Autodesk Inventor part; units mm, degrees
ref_plane "YZ Plane" through (0, 0, 0) normal (1, 0, 0) x (0, 1, 0)
ref_plane "XZ Plane" through (0, 0, 0) normal (0, 1, 0) x (-1, 0, 0)
ref_plane "XY Plane" through (0, 0, 0) normal (0, 0, 1) x (1, 0, 0)
sketch "Sketch1" plane through (0, 0, 0) normal (0, 1, 0) x (-1, 0, 0)
  line L0 (0, 0) -> (-30.566, 0)
  line L1 (-30.566, 0) -> (-30.566, -53)
  line L2 (-30.566, -53) -> (0, -53)
  line L3 (0, -53) -> (0, 0)
  dimension "d0" = 30.566
  dimension "d1" = 53
extrude "Extrusion1" add sketch "Sketch1" along normal blind 2
ref_plane "Work Plane1" through (30.566, 0, -23) normal (0, 0, -1) x (-1, 0, 0)
sketch "Sketch2" plane through (30.566, 0, -23) normal (0, 0, -1) x (-1, 0, 0)
  point P0 (30.566, 0)
sketch "Sketch3" plane through (30.566, 0, -53) normal (0, 0, -1) x (-1, 0, 0)
  circle A0 centre (30.566, 0) radius 1
  circle A1 centre (30.566, 0) radius 2
  line L0 (30.566, -2) -> (15.283, 0)
  line L1 (15.283, 0) -> (28.566, 0)
  line L2 (0, 0) -> (30.566, 0)
  dimension "d5" = 2
  dimension "d6" = 4
extrude "Extrusion2" add sketch "Sketch3" against normal blind 53 contours A1 L0 | A1 L0 L1 picked at (30.3543, -1.6418)
sketch "Sketch4" plane through (30.566, 0, -53) normal (0, 0, -1) x (-1, 0, 0)
  arc A0 (29.566, 0) -> (30.566, 1) centre (30.566, 0) ccw
  circle A1 centre (30.566, 0) radius 1
  point P0 (30.566, 1)
extrude "Extrusion3" cut sketch "Sketch4" against normal blind 53
chamfer "Chamfer2" distance 2 angle 45 1 edges at (30.566, 0, -26.5)
equation "\"BendRadius\" = Thickness"
equation "\"BendReliefWidth\" = Thickness"
equation "\"BendReliefDepth\" = 0.5 * Thickness"
equation "\"CornerReliefSize\" = 4 * Thickness"
equation "\"MinimumRemnant\" = 2 * Thickness"
equation "\"TransitionRadius\" = BendRadius"
equation "\"JacobiRadiusSize\" = BendRadius"
equation "\"GapSize\" = Thickness"
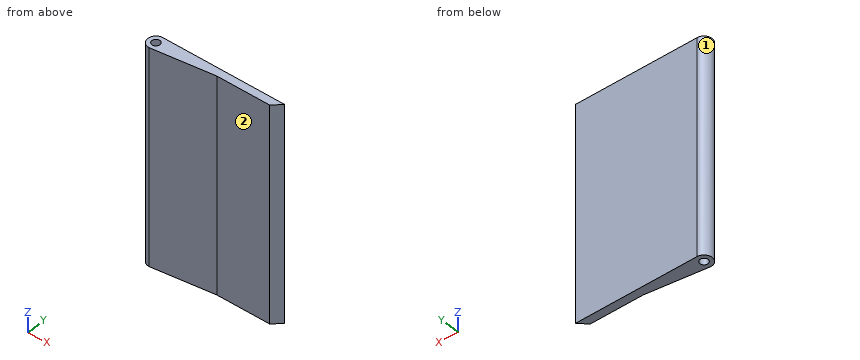
Here's how the part is built. I have some questions about the finished solid (model axes, mm). Face numbers are marked on the shaded views. A direction names the side the tool comes from. Give positions to 0.01 mm unless a question says otherwise; leave off trailing zeros. Write each loop counter-clockwise with the first axis right and the second up, starting at its lowest first coordinate (ties: lowest second). Pieces come first, ordered by that corner, then holes. Notation, with made-up numbers: (8, 29) -> (55, 29) arc R21 cw to (55, 61) -> close; hole circle Ø4 at (79.25, 63). An arc over 180 degrees is marked (long way). Use one line per item in the form item = value.
1) I'm going to push flat-ended pins straight in: pin 1 (10 mm diameter, centred on x = 16, z = -26.5, fed in from -Y); pin 2 (3 mm diameter, centred on x = 9, z = -5.5, fed in from -Y); pin 3 (4 mm diameter, centred on x = 14.5, z = -19, fed in from -Y). Where does each tip first touch, or does it pass through?
Verdict:
pin_1 = -0.56
pin_2 = -1.02
pin_3 = -0.36
2) On a 3-axis mill with a long thin cutter (end or side, diameter ignored), from which of +Z, -Z, +X, -X, +Y, -Y can I reach the whole of each face in a straight line? I mean the marked faces 1 and 2. Say none if no direction works.
Verdict:
face_1 = +Z, -Z, -X
face_2 = +Z, -Z, +X, -Y
3) If I drill on L1, parallel to Y at x = 0, z = -32; L2, parallel to Y at x = 26, z = -17; L3, parallel to Y at x = 11, z = -2.5, over which ranges is the centre line in solid material (lowest first)? Write a range as [from, to].
Verdict:
L1 = [-2, -1], [1, 2]
L2 = [0, 2]
L3 = [-0.56, 2]
4) Suppose I cut it at B-B (x = 4.5). Please give me the cut outline in (y, z).
Verdict:
outline = (-1.41, -53) -> (2, -53) -> (2, 0) -> (-1.41, 0) -> close
